Can you work these out from the model? Positions are in its coordinate system, mm. A direction names the side the tool comes from. Give positions to 0.01 mm unless a question says otherwise; leave off trailing zeros. Loops run counter-clockwise (first coordinate to the right, second up) from the corner with the lowest first, then second, coordinate; pieces in that order, holes last. Notation, with made-up numbers: (58, 77.25) - (80, 77.25) arc R17 cw to (80, 108.25) - close; hole circle Ø4 at (78, -33.75). An arc over 180 degrees is marked (long way). Answer as a JSON object with one key per item and string values.
```python
from build123d import *

# Parameters (mm, degrees)
EXTRUDE_1_DEPTH     = 6
SKETCH_3_R          = 3
EXTRUDE_2_DEPTH     = 5.5
SKETCH_4_R          = 2.5
EXTRUDE_3_DEPTH     = 5
SKETCH_5_R          = 5.05
CUT_EXTRUDE_1_DEPTH = 4
SKETCH_6_R          = 4
CUT_EXTRUDE_2_DEPTH = 3
SKETCH_7_R          = 7.55
CUT_EXTRUDE_3_DEPTH = 4
SKETCH_8_R          = 6
CUT_EXTRUDE_4_DEPTH = 3
FILLET_1_R          = 3
EXTRUDE_4_DEPTH     = 6
SKETCH_10_R         = 1.6
CUT_EXTRUDE_5_DEPTH = 17.5
SKETCH_11_R         = 2.1
CUT_EXTRUDE_6_DEPTH = 6
FILLET_2_R          = 5


with BuildPart() as part:
    # 草图1 → 凸台-拉伸1 (new body)
    with BuildSketch(Plane.XY):
        with BuildLine():
            Line((-24, 0), (-24, -45))
            Line((-24, -45), (24, -45))
            Line((24, -45), (24, 0))
            ThreePointArc((24, 0), (0, 24), (-24, 0))
        make_face()
    extrude(amount=EXTRUDE_1_DEPTH)

    # 草图3 → 凸台-拉伸2 (add)
    with BuildSketch(Plane.XY.offset(6)):
        with Locations((-15, 6.899039913)):
            Circle(SKETCH_3_R)
        with Locations((15, 6.899039913)):
            Circle(SKETCH_3_R)
    extrude(amount=EXTRUDE_2_DEPTH)

    # 草图4 → 凸台-拉伸3 (add)
    with BuildSketch(Plane.XY.offset(11.5)):
        with Locations((-15, 6.899039913)):
            Circle(SKETCH_4_R)
        with Locations((15, 6.899039913)):
            Circle(SKETCH_4_R)
    extrude(amount=EXTRUDE_3_DEPTH)

    # 草图5 → 切除-拉伸1 (cut)
    with BuildSketch(Plane.XY.offset(6)):
        with Locations((1.743114855, -8.076106038)):
            Circle(SKETCH_5_R)
    extrude(amount=-CUT_EXTRUDE_1_DEPTH, mode=Mode.SUBTRACT)

    # 草图6 → 切除-拉伸2 (cut, through all)
    with BuildSketch(Plane.XY.offset(2)):
        with Locations((1.743114855, -8.076106038)):
            Circle(SKETCH_6_R)
    extrude(amount=-CUT_EXTRUDE_2_DEPTH, mode=Mode.SUBTRACT)

    # 草图7 → 切除-拉伸3 (cut)
    with BuildSketch(Plane.XY.offset(6)):
        with Locations((0, -28)):
            Circle(SKETCH_7_R)
    extrude(amount=-CUT_EXTRUDE_3_DEPTH, mode=Mode.SUBTRACT)

    # 草图8 → 切除-拉伸4 (cut, through all)
    with BuildSketch(Plane.XY.offset(2)):
        with Locations((0, -28)):
            Circle(SKETCH_8_R)
    extrude(amount=-CUT_EXTRUDE_4_DEPTH, mode=Mode.SUBTRACT)

    # 圆角1
    fillet_1_edges = [part.edges().sort_by_distance(p)[0] for p in [
        (-18, 6.899039913, 6),
        (12, 6.899039913, 6),
    ]]
    fillet(fillet_1_edges, radius=FILLET_1_R)

    # 草图9 → 凸台-拉伸4 (add)
    with BuildSketch(Plane.XY.offset(6)):
        with BuildLine():
            Line((24, -45), (24, -8.109291107))
            ThreePointArc((24, -8.109291107), (21.638033238, -9.293134578), (19.124765434, -10.107908964))
            ThreePointArc((19.124765434, -10.107908964), (15.930250057, -18.32184636), (9.137474346, -23.93717308))
            ThreePointArc((9.137474346, -23.93717308), (-0.871557427, -37.961946981), (-8.293153088, -22.412190782))
            ThreePointArc((-8.293153088, -22.412190782), (-13.156547867, -17.254888679), (-15.575163477, -10.591505733))
            ThreePointArc((-15.575163477, -10.591505733), (-19.945835244, -9.887523575), (-24, -8.109291107))
            Line((-24, -8.109291107), (-24, -45))
            Line((-24, -45), (24, -45))
        make_face()
    extrude(amount=EXTRUDE_4_DEPTH)

    # 草图10 → 切除-拉伸5 (cut, through all)
    with BuildSketch(Plane(origin=(0, 0, 0), x_dir=(-1, 0, 0), z_dir=(0, 0, -1))):
        with Locations((-20, -39)):
            Circle(SKETCH_10_R)
        with Locations((-20, -17)):
            Circle(SKETCH_10_R)
        with Locations((20, -39)):
            Circle(SKETCH_10_R)
        with Locations((20, -17)):
            Circle(SKETCH_10_R)
    extrude(amount=-CUT_EXTRUDE_5_DEPTH, mode=Mode.SUBTRACT)

    # 草图11 → 切除-拉伸6 (cut)
    with BuildSketch(Plane(origin=(0, 0, 0), x_dir=(-1, 0, 0), z_dir=(0, 0, -1))):
        with Locations((-20, -17)):
            Circle(SKETCH_11_R)
        with Locations((-20, -39)):
            Circle(SKETCH_11_R)
        with Locations((20, -17)):
            Circle(SKETCH_11_R)
        with Locations((20, -39)):
            Circle(SKETCH_11_R)
    extrude(amount=-CUT_EXTRUDE_6_DEPTH, mode=Mode.SUBTRACT)

    # 圆角2
    fillet_2_edges = [part.edges().sort_by_distance(p)[0] for p in [
        (24, -45, 6),
        (-24, -45, 6),
    ]]
    fillet(fillet_2_edges, radius=FILLET_2_R)


solid = part.part
```
1) I'm going to push flat-ended pins straight in: P1, Ø2, axis at y = -14.5, z = 14.5, coming from the -X side; P2, Ø1.5, axis at x = -8, z = 9.5, coming from the +Y side; P3, Ø10, axis at x = -9, y = -26.5, coming from the +Z side; P4, Ø7.5, axis at x = -3, y = -31, coming from the +Z side. Where does each tip first touch, or does it pass through?
Check sheet entries:
{"P1": "through", "P2": "y = -22.08", "P3": "z = 12", "P4": "z = 6"}
2) Imagine slicing it at C-C on y = -17. Write out the boundary of the cut face in (x, z), and give its area (3 significant figures).
Check sheet entries:
{"outline": "(-24, 0) - (-22.1, 0) - (-22.1, 6) - (-21.6, 6) - (-21.6, 12) - (-24, 12) - close; (-18.4, 6) - (-17.9, 6) - (-17.9, 0) - (17.9, 0) - (17.9, 6) - (18.4, 6) - (18.4, 12) - (16.8, 12) - (16.8, 6) - (-13.31, 6) - (-13.31, 12) - (-18.4, 12) - close; (21.6, 6) - (22.1, 6) - (22.1, 0) - (24, 0) - (24, 12) - (21.6, 12) - close", "area": "307 mm2"}
3) Imagine slicing it at B-B on z = 10.5. Write out the boundary of the cut face in (x, y), and give its area (3 significant figures).
Check sheet entries:
{"outline": "(-24, -40) arc R5 ccw to (-19, -45) - (19, -45) arc R5 ccw to (24, -40) - (24, -8.11) arc R17.5 cw to (19.12, -10.11) arc R17.5 cw to (9.14, -23.94) arc R10 cw (long way) to (-8.29, -22.41) arc R17.5 cw to (-15.58, -10.59) arc R17.5 cw to (-24, -8.11) - close; circle Ø6 at (-15, 6.9); circle Ø6 at (15, 6.9); hole circle Ø3.2 at (-20, -39); hole circle Ø3.2 at (-20, -17); hole circle Ø3.2 at (20, -39); hole circle Ø3.2 at (20, -17)", "area": "1,060 mm2"}
4) Imagine slicing it at D-D on z = 4.5. Write out the boundary of the cut face in (x, y), and give its area (3 significant figures).
Check sheet entries:
{"outline": "(-24, -40) arc R5 ccw to (-19, -45) - (19, -45) arc R5 ccw to (24, -40) - (24, 0) arc R24 ccw to (-24, 0) - close; hole circle Ø4.2 at (-20, -39); hole circle Ø4.2 at (-20, -17); hole circle Ø15.1 at (0, -28); hole circle Ø10.1 at (1.74, -8.08); hole circle Ø4.2 at (20, -39); hole circle Ø4.2 at (20, -17)", "area": "2,740 mm2"}
5) Which directions (+Z, -Z, +X, -X, +Y, -Y) give clear straight access to the entire face, cutting with the end or side of a thin tool? Please do faces 1 (the cylindrical face through (20.35, -40.56, 8.96)), 2 (the cylindrical face through (19.031, -40.863, 2.958)), 3 (the cylindrical face through (16.003, -18.22, 8.958)).
Check sheet entries:
{"face 1": "+Z, -Z", "face 2": "-Z", "face 3": "+Z"}
6) If we mould it in two halves opening along Y, with no side actions, what happens to faces 4 (the cylindrical face through (23, -43, 6)), 5 (the cylindrical face through (-17.21, 8.93, 10.23)), 6 (the flat face through (-24, -20, 6))? For each: released by +Y, released by -Y, zero draft, split by the parting line, or undercut.
Check sheet entries:
{"face 4": "released by -Y", "face 5": "undercut", "face 6": "zero draft"}
7) Imagine slicing it at A-A on x = 0.5. Write out the boundary of the cut face in (y, z).
Check sheet entries:
{"outline": "(-45, 0) - (-33.98, 0) - (-33.98, 2) - (-35.53, 2) - (-35.53, 6) - (-37.99, 6) - (-37.99, 12) - (-45, 12) - close; (-22.02, 0) - (-11.88, 0) - (-11.88, 2) - (-12.97, 2) - (-12.97, 6) - (-20.47, 6) - (-20.47, 2) - (-22.02, 2) - close; (-4.27, 0) - (23.99, 0) - (23.99, 6) - (-3.18, 6) - (-3.18, 2) - (-4.27, 2) - close"}
8) I need wall thicknesses on L1, parallel to Y at x = 20, z = 2.55; L2, parallel to X at y = -16, z = 3.25; L3, parallel to Z at x = 1, y = 7. Which ranges of each line are inside material? Lowest first, please.
Check sheet entries:
{"L1": "-44.9 to -41.1, -36.9 to -19.1, -14.9 to 13.27", "L2": "-24 to -21.85, -18.15 to 18.15, 21.85 to 24", "L3": "0 to 6"}
